Here's how the part is built. I have some questions about the finished solid (model axes, mm). A direction names the side the tool comes from. Round coordinates to 2 decimals unless told otherwise and drop trailing zeros. Order: outer loops, then holes, each group sorted by start corner. A loop starts at its lowest first (then second) coordinate and runs counter-clockwise, first axis right, second up. Notation, with made-up numbers: (-29.75, 78.25) -> (0.25, 78.25) arc R24 ccw to (0.25, 112.25) -> close; hole circle Ø11 at (7.5, 61.25). An arc over 180 degrees is marked (long way). One line per item, written item: value.
Autodesk Inventor part; units mm, degrees
ref_plane "YZ Plane" through (0, 0, 0) normal (1, 0, 0) x (0, 1, 0)
ref_plane "XZ Plane" through (0, 0, 0) normal (0, 1, 0) x (-1, 0, 0)
ref_plane "XY Plane" through (0, 0, 0) normal (0, 0, 1) x (1, 0, 0)
sketch "Sketch1" plane through (0, 0, 0) normal (1, 0, 0) x (0, 1, 0)
  line L0 (12.5, 0) -> (-12.5, 0)
  line L1 (12.5, 0) -> (12.5, 3.5)
  line L2 (15.5, 6.5) -> (17.5, 6.5)
  line L3 (-12.5, 0) -> (-12.5, 3.5)
  line L4 (-15.5, 6.5) -> (-17.5, 6.5)
  line L5 (17.5, 5.5) -> (15.5, 5.5)
  line L6 (13.5, 3.5) -> (13.5, -1)
  line L7 (13.5, -1) -> (-13.5, -1)
  line L8 (-13.5, -1) -> (-13.5, 3.5)
  line L9 (-15.5, 5.5) -> (-17.5, 5.5)
  line L10 (17.5, 5.5) -> (17.5, 6.5)
  line L11 (-17.5, 5.5) -> (-17.5, 6.5)
  arc A0 (15.5, 5.5) -> (13.5, 3.5) centre (15.5, 3.5) ccw
  arc A1 (15.5, 6.5) -> (12.5, 3.5) centre (15.5, 3.5) ccw
  arc A2 (-12.5, 3.5) -> (-15.5, 6.5) centre (-15.5, 3.5) ccw
  arc A3 (-13.5, 3.5) -> (-15.5, 5.5) centre (-15.5, 3.5) ccw
  point P0 (0, 0)
  point P1 (0, 0)
  dimension "d0" = 25
  dimension "d2" = 1
  dimension "d3" = 35
  dimension "d4" = 2
  dimension "d5" = 2
  dimension "d6" = 7.5
extrude "Extrusion1" add sketch "Sketch1" along normal blind 200
sketch "Sketch2" plane through (0, -12.5, 0) normal (0, 0, 1) x (1, 0, 0)
  line L0 (10, 12.5) -> (25, 12.5) construction
  line L1 (10, 9.5) -> (25, 9.5)
  line L2 (25, 15.5) -> (10, 15.5)
  arc A0 (10, 15.5) -> (10, 9.5) centre (10, 12.5) ccw
  arc A1 (25, 9.5) -> (25, 15.5) centre (25, 12.5) ccw
  line L3 (0, 25) -> (0, 0)
  point P0 (0, 12.5)
  point P1 (17.5, 12.5)
  point P2 (0, 12.5)
  dimension "d9" = 15
  dimension "d10" = 6
  dimension "d11" = 10
extrude "Extrusion2" cut sketch "Sketch2" against normal through all
pattern_linear "Rectangular Pattern1" count 10 spacing 30 along (1, 0, 0) of "Extrusion2"
equation "\"d12\" = d9"
properties part number "din_rail" material "Aluminum 6061"
Q1. For P1, Ø0.8, axis at x = 197, z = -0.5, coming from the +Y side; P2, Ø3, axis at x = 117.5, z = 1.5, coming from the -Y side; P3, Ø12.5, axis at x = 95, y = 5.5, coming from the +Z side, each with a flat end and sliding along its axis, tell me the tip position at first contact or that it passes through.
Answers:
P1: y = 13.5
P2: y = -13.5
P3: z = 0
Q2. If we mould it in two halves opening along Y, with no side actions, what happens to faces 1 (the face through (99, 13.5, 1)), 2 (the face through (99, 3, 0)), 3 (the face through (99, -13.5, 1)), 4 (the face through (200, 10.8, -0.3))? For each: pulls with the +Y half, pulls with the -Y half, needs draft (parallel to the pull), parting line crosses it, or undercut.
Answers:
face 1: pulls with the +Y half
face 2: undercut
face 3: pulls with the -Y half
face 4: needs draft
Q3. I want a section at A-A on z = 2. Write out the boundary of the cut face in (x, y).
Answers:
outline: (0, -13.5) -> (200, -13.5) -> (200, -12.5) -> (0, -12.5) -> close; (0, 12.5) -> (200, 12.5) -> (200, 13.5) -> (0, 13.5) -> close
Q4. I want a section at C-C on y = 0. Write out the boundary of the cut face in (x, z), then the cut area to 3 significant figures.
Answers:
outline: (0, -1) -> (7, -1) -> (7, 0) -> (0, 0) -> close; (28, -1) -> (37, -1) -> (37, 0) -> (28, 0) -> close; (58, -1) -> (67, -1) -> (67, 0) -> (58, 0) -> close; (88, -1) -> (97, -1) -> (97, 0) -> (88, 0) -> close; (118, -1) -> (127, -1) -> (127, 0) -> (118, 0) -> close; (148, -1) -> (157, -1) -> (157, 0) -> (148, 0) -> close; (178, -1) -> (187, -1) -> (187, 0) -> (178, 0) -> close
area: 61.0 mm2
Q5. Which directions (+Z, -Z, +X, -X, +Y, -Y) give clear straight access to the entire face, cutting with the end or side of a thin tool? Please do faces 5 (the face through (0, -0.1, -0.6)), 6 (the face through (99, -12.5, 2)).
Answers:
face 5: +Z, -Z, -X, +Y, -Y
face 6: +Z, +X, -X
Q6. I need wall thicknesses on line 1 along Y through (x, z) = (182, 3.5); line 2 along Z through (x, y) = (76.5, -7.5); line 3 along Y through (x, z) = (90.5, 4.5). Which ranges of each line are inside material? Lowest first, please.
Answers:
line 1: -13.5 to -12.5, 12.5 to 13.5
line 2: -1 to 0
line 3: -13.77 to -12.67, 12.67 to 13.77
Q7. I want a section at B-B on x = 169. Write out the boundary of the cut face in (y, z).
Answers:
outline: (-17.5, 5.5) -> (-15.5, 5.5) arc R2 cw to (-13.5, 3.5) -> (-13.5, -1) -> (-3, -1) -> (-3, 0) -> (-12.5, 0) -> (-12.5, 3.5) arc R3 ccw to (-15.5, 6.5) -> (-17.5, 6.5) -> close; (3, -1) -> (13.5, -1) -> (13.5, 3.5) arc R2 cw to (15.5, 5.5) -> (17.5, 5.5) -> (17.5, 6.5) -> (15.5, 6.5) arc R3 ccw to (12.5, 3.5) -> (12.5, 0) -> (3, 0) -> close
